Geometry check sheet. Reference: the model listing, model coordinates, mm. A direction names the side the tool comes from. Coordinates: 2 decimals unless noted, no trailing zeros. Loops run counter-clockwise (first coordinate to the right, second up) from the corner with the lowest first, then second, coordinate; pieces in that order, holes last.
from build123d import *

# Parameters (mm, degrees)
SKETCH3_R           = 17.8816
BOSS_EXTRUDE2_DEPTH = 0.762
DOME1_FACE_RADIUS   = 17.8816
DOME1_HEIGHT        = 12.192
SKETCH4_R           = 4.191
CUT_EXTRUDE1_DEPTH  = 1.016
SKETCH5_R           = 17.3736
CUT_EXTRUDE2_DEPTH  = 1.27


# Read off the part's stored shape, not the designer's step: Shell3
with BuildPart() as part:
    # Sketch3 → Boss-Extrude2 (new body)
    with BuildSketch(Plane.XY):
        with Locations(Location((0, 0, 0), (0, 0, 180))):
            Circle(SKETCH3_R)
    extrude(amount=BOSS_EXTRUDE2_DEPTH)

    # Dome1: a dome of height H over a round flat face of radius A is a cap of a sphere of radius (A * A + H * H) / (2 * H)
    dome1_r = (DOME1_FACE_RADIUS * DOME1_FACE_RADIUS + DOME1_HEIGHT * DOME1_HEIGHT) / (2 * DOME1_HEIGHT)
    dome1_base = Plane((0, 0, 0.762), z_dir=(0, 0, 1))
    with Locations(dome1_base.offset(DOME1_HEIGHT - dome1_r)):
        dome1_ball = Sphere(dome1_r, mode=Mode.PRIVATE)
    add(split(dome1_ball, bisect_by=dome1_base, keep=Keep.TOP, mode=Mode.PRIVATE))

    # Sketch4 → Cut-Extrude1 (cut)
    with BuildSketch(Plane.XY.offset(12.192)):
        Circle(SKETCH4_R)
    extrude(amount=CUT_EXTRUDE1_DEPTH, mode=Mode.SUBTRACT)

    # Sketch5 → Cut-Extrude2 (cut)
    with BuildSketch(Plane(origin=(0, 0, 0), x_dir=(-1, 0, 0), z_dir=(0, 0, -1))):
        Circle(SKETCH5_R)
    extrude(amount=-CUT_EXTRUDE2_DEPTH, mode=Mode.SUBTRACT)

    # Shell3 outline → Shell3 (revolve, cut)
    with BuildSketch(Plane.XZ):
        with BuildLine():
            ThreePointArc((17.120328578, 1.269999983), (12.123689074, 7.983859192), (4.698999991, 11.846022294))
            Line((4.698999991, 11.846022294), (4.699, 11.684))
            Line((4.699, 11.684), (0, 11.684))
            Line((0, 11.684), (0, 1.269999983))
            Line((0, 1.269999983), (17.120328578, 1.269999983))
        make_face()
    revolve(axis=Axis((0, 0, 0), (0, 0, 1)), mode=Mode.SUBTRACT)


solid = part.part
(1) Sectioned sample at B-B on x = 3.5. Record the cut outline in (y, z).
Findings:
outline: (-17.54, 0) - (-17.02, 0) - (-17.02, 1.27) - (-16.76, 1.27) arc R18.37 cw to (-3.14, 11.85) - (-3.14, 11.68) - (3.14, 11.68) - (3.14, 11.85) arc R18.37 cw to (16.76, 1.27) - (17.02, 1.27) - (17.02, 0) - (17.54, 0) - (17.54, 0.76) arc R18.89 ccw to (2.31, 12.49) - (2.31, 12.19) - (-2.31, 12.19) - (-2.31, 12.49) arc R18.89 ccw to (-17.54, 0.76) - close
(2) Sectioned sample at D-D on z = 3. Record the cut outline in (x, y).
Findings:
outline: circle Ø33.67 at (0, 0); hole circle Ø32.5 at (0, 0)
(3) Draft check along X on faces 3 (the cylindrical face through (3.876, 17.456, 0.376)), 4 (the cylindrical face through (3.77, -16.96, 0.63)). Enter one of: +X half, -X half, draft (parallel to the pull), parting line (faces both ways), or undercut.
Findings:
face 3: parting line
face 4: undercut
(4) Gauge pin test, flat ends, axial feed: pin 1 Ø5 at (x, y) = (-11.5, 8) entering from -Z; pin 2 Ø1 at (x, z) = (5, 4) entering from +Y; pin 3 Ø2 at (x, y) = (12.5, -6) entering from -Z. Record the tip position at first contact, or that the pin passes through.
Findings:
pin 1: stops at z = 2.53
pin 2: stops at y = 15.81
pin 3: stops at z = 5.09
(5) Sectioned sample at C-C on y = 12. Record the cut outline in (x, z).
Findings:
outline: (-13.26, 0) - (-12.56, 0) - (-12.56, 1.27) - (-12.21, 1.27) arc R14.34 cw to (12.21, 1.27) - (12.56, 1.27) - (12.56, 0) - (13.26, 0) - (13.26, 0.76) arc R15 ccw to (-13.26, 0.76) - close
(6) Sectioned sample at A-A on y = 0. Record the cut outline in (x, z), and give its area (3 significant figures).
Findings:
outline: (-17.88, 0) - (-17.37, 0) - (-17.37, 1.27) - (-17.12, 1.27) arc R18.7 cw to (-4.7, 11.85) - (-4.7, 11.68) - (4.7, 11.68) - (4.7, 11.85) arc R18.7 cw to (17.12, 1.27) - (17.37, 1.27) - (17.37, 0) - (17.88, 0) - (17.88, 0.76) arc R19.21 ccw to (4.19, 12.49) - (4.19, 12.19) - (-4.19, 12.19) - (-4.19, 12.49) arc R19.21 ccw to (-17.88, 0.76) - close
area: 23.8 mm2
(7) Scan lines: L1, parallel to Y at x = 0, z = 0.4; L2, parallel to Y at x = -7.5, z = 8.5; L3, parallel to X at y = 6, z = 1. Record each from-to range of solid material in increasing order.
Findings:
L1: y = -17.88 to -17.37, 17.37 to 17.88
L2: y = -9.75 to -8.7, 8.7 to 9.75
L3: x = -16.74 to -16.3, 16.3 to 16.74
(8) Access from +Z, -Z, +X, -X, +Y, -Y to the whole of each face (thin tool, end or side, straight path). Record for faces 1 (the flat face through (0, 0, 12.192)), 2 (the flat face through (0, 0, 11.684)).
Findings:
face 1: +Z
face 2: -Z
